The figure shows three views and two pictorial views of one solid part (mm, origin at its lowest corner). Answer the questions. Round coordinates to 2 decimals unless told otherwise and drop trailing zeros. Order: outer loops, then holes, each group sorted by start corner. A loop starts at its lowest first (then second) coordinate and runs counter-clockwise, first axis right, second up. Notation, with made-up numbers: (84.25, 14) -> (101.25, 14) arc R24 ccw to (101.25, 36) -> close; hole circle Ø3 at (-32, -13.75). An arc over 180 degrees is marked (long way). Return JSON: item names as keys, results as strings. Group by question number.
(1) The part is cut by section B-B (y = 184). Determine the outline of the cut face in (x, z), plus the area to 3 significant figures.
(2) The part is cut by section D-D (x = 432). Determine the outline of the cut face in (y, z).
(3) The part is cut by section C-C (z = 5.5). Determine the outline of the cut face in (x, y), plus the area to 3 significant figures.
(4) Consider line 1 (X direction, y = 176, z = 22.5); line 2 (Z direction, x = 207.5, y = 219); line 3 (Y direction, x = 163, z = 10.75). Determine where each line is inside the solid, lowest interval first. Write a range as [from, to].
(5) Determine the mould class of the marked faces 1 and 2 for opening direction X: +X half, -X half, draft (parallel to the pull), parting line (faces both ways), or undercut.
(6) The part is cut by section A-A (x = 555.5). Determine the outline of the cut face in (y, z), plus the area to 3 significant figures.
(7) Each of these flat-tipped pins is pushed along its axis until it touches: pin 1 (19 mm diameter, centred on x = 26.5, y = 130, fed in from +Z); pin 2 (3 mm diameter, centred on x = 286.5, z = 16, fed in from -Y); pin 3 (9.5 mm diameter, centred on x = 568, y = 273.5, fed in from -Z); pin 4 (10 mm diameter, centred on x = 321, z = 8, fed in from +Y). Where does it stop, or does it pass through?
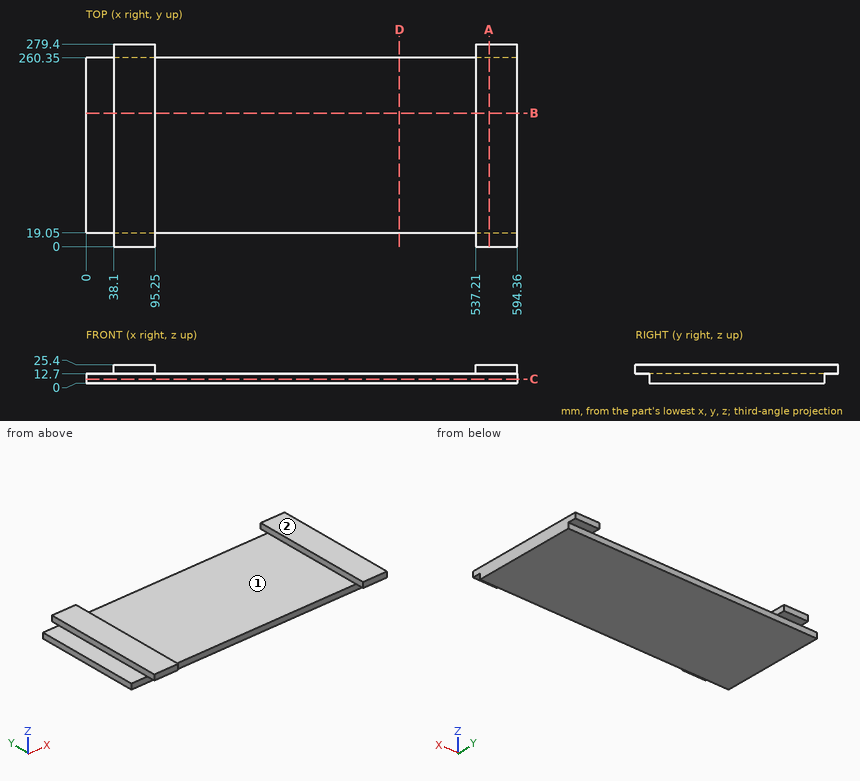
Answer below:
{
 "1": {"outline": "(0, 0) -> (594.36, 0) -> (594.36, 25.4) -> (537.21, 25.4) -> (537.21, 12.7) -> (95.25, 12.7) -> (95.25, 25.4) -> (38.1, 25.4) -> (38.1, 12.7) -> (0, 12.7) -> close", "area": "9,000 mm²"},
 "2": {"outline": "(19.05, 0) -> (260.35, 0) -> (260.35, 12.7) -> (19.05, 12.7) -> close"},
 "3": {"outline": "(0, 19.05) -> (594.36, 19.05) -> (594.36, 260.35) -> (0, 260.35) -> close", "area": "143,000 mm²"},
 "4": {"line 1": "x = [38.1, 95.25], [537.21, 594.36]", "line 2": "z = [0, 12.7]", "line 3": "y = [19.05, 260.35]"},
 "5": {"face 1": "undercut", "face 2": "draft"},
 "6": {"outline": "(0, 12.7) -> (19.05, 12.7) -> (19.05, 0) -> (260.35, 0) -> (260.35, 12.7) -> (279.4, 12.7) -> (279.4, 25.4) -> (0, 25.4) -> close", "area": "6,610 mm²"},
 "7": {"pin 1": "stops at z = 12.7", "pin 2": "passes through", "pin 3": "stops at z = 12.7", "pin 4": "stops at y = 260.35"}
}
